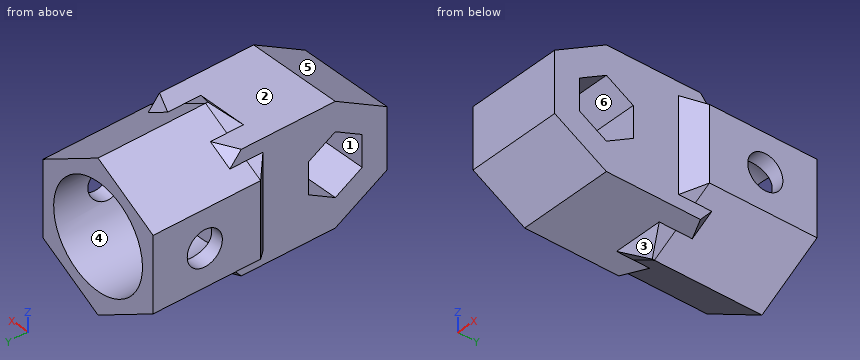
```python
from build123d import *

# Parameters (mm, degrees)
SALIENTE_EXTRUIR1_DEPTH      = 4.6
SALIENTE_EXTRUIR1_DEPTH_BACK = 4.6
SALIENTE_EXTRUIR2_START      = 4
CROQUIS2_R                   = 5
SALIENTE_EXTRUIR2_DEPTH      = 10
CROQUIS4_W                   = 9.2
CROQUIS4_H                   = 2.771281292
SALIENTE_EXTRUIR3_DEPTH      = 9
SALIENTE_EXTRUIR4_START      = 2.6
CROQUIS4_3_W                 = 9.2
CROQUIS4_3_H                 = 6.0044428
SALIENTE_EXTRUIR4_DEPTH      = 6.4
SALIENTE_EXTRUIR5_START      = 3.6
CROQUIS2_2_R                 = 5
SALIENTE_EXTRUIR5_DEPTH      = 0.4
CHAFL_N1_SIZE                = 1.2
CHAFL_N2_SIZE                = 1.6
CROQUIS5_R                   = 1.7
CORTAR_EXTRUIR1_DEPTH        = 24.791034726


with BuildPart() as part:
    # Croquis1 → Saliente-Extruir1 (new, two sides: drawn at the far end of the back side and taken through both)
    with BuildSketch(Plane(origin=(0, 0, 0), x_dir=(0, 0, -1), z_dir=(1, 0, 0)).offset(-SALIENTE_EXTRUIR1_DEPTH_BACK)):
        Polygon((2.886751346, 5), (-2.886751346, 5), (-5.773502692, 0), (-2.886751346, -5), (2.886751346, -5), (5.773502692, 0), align=None)
        Polygon((3.0022214, 0), (1.5011107, 2.6), (-1.5011107, 2.6), (-3.0022214, 0), (-1.5011107, -2.6), (1.5011107, -2.6), align=None, mode=Mode.SUBTRACT)
    extrude(amount=SALIENTE_EXTRUIR1_DEPTH + SALIENTE_EXTRUIR1_DEPTH_BACK)



with BuildPart() as body_2:
    # Croquis2 → Saliente-Extruir2 (new body)
    with BuildSketch(Plane(origin=(0, 5, 0), x_dir=(1, 0, 0), z_dir=(0, 1, 0)).offset(SALIENTE_EXTRUIR2_START)):
        Polygon((0, 7.159143338), (-6.2, 3.579571669), (-6.2, -3.579571669), (0, -7.159143338), (6.2, -3.579571669), (6.2, 3.579571669), align=None)
        with Locations(Location((0, 0, 0), (0, 0, 270))):
            Circle(CROQUIS2_R, mode=Mode.SUBTRACT)
    extrude(amount=SALIENTE_EXTRUIR2_DEPTH)


with BuildPart() as part_1:
    add(part.part)

    add(body_2.part)  # Saliente-Extruir3 merges body 2
    # Croquis4 → Saliente-Extruir3 (add)
    with BuildSketch(Plane(origin=(0, 0, 0), x_dir=(1, 0, 0), z_dir=(0, 1, 0))):
        with Locations((0, -4.387862046)):
            Rectangle(CROQUIS4_W, CROQUIS4_H)
        with Locations((0, 4.387862046)):
            Rectangle(CROQUIS4_W, CROQUIS4_H)
    extrude(amount=SALIENTE_EXTRUIR3_DEPTH)

    # Croquis4<3> → Saliente-Extruir4 (add)
    with BuildSketch(Plane(origin=(0, 0, 0), x_dir=(1, 0, 0), z_dir=(0, 1, 0)).offset(SALIENTE_EXTRUIR4_START)):
        Rectangle(CROQUIS4_3_W, CROQUIS4_3_H)
    extrude(amount=SALIENTE_EXTRUIR4_DEPTH)

    # Croquis2<2> → Saliente-Extruir5 (add)
    # profile 1 of 2: a face of its own
    with BuildSketch(Plane(origin=(0, 5, 0), x_dir=(1, 0, 0), z_dir=(0, 1, 0)).offset(SALIENTE_EXTRUIR5_START)):
        Polygon((6.2, -3.579571669), (6.2, 3.579571669), (0, 7.159143338), (-6.2, 3.579571669), (-6.2, -3.579571669), (0, -7.159143338), align=None)
        with Locations(Location((0, 0, 0), (0, 0, 270))):
            Circle(CROQUIS2_2_R, mode=Mode.SUBTRACT)
    # profile 2 of 2: a face of its own
    with BuildSketch(Plane(origin=(0, 5, 0), x_dir=(1, 0, 0), z_dir=(0, 1, 0)).offset(SALIENTE_EXTRUIR5_START)):
        with Locations(Location((0, 0, 0), (0, 0, 270))):
            Circle(CROQUIS2_2_R)
    extrude(amount=SALIENTE_EXTRUIR5_DEPTH)

    # Chaflán1
    # the kernel refuses this chamfer: 1.2 mm, written as the material it adds along each edge
    with BuildSketch(Plane(origin=(-0.272571358, 9, 7.316512485), x_dir=(0.49981095845564805, -0.027495876610585935, 0.8656979742248805), z_dir=(0.8660254037844388, 0, -0.49999999999999967))) as chafl_n1_piece_1_section:
        Polygon((CHAFL_N1_SIZE * 0.999621916911, -CHAFL_N1_SIZE * 0.0274958766106), (-CHAFL_N1_SIZE * 0.0274958766106, -CHAFL_N1_SIZE * 0.999621916911), (0, 0), align=None)
    chafl_n1_piece_1 = extrude(amount=8.712380356, mode=Mode.PRIVATE)
    chafl_n1_piece_1 = split(chafl_n1_piece_1, bisect_by=Plane(origin=(4.6, 9.457, 5.303539573), z_dir=(-1, 0, 0)), keep=Keep.TOP, mode=Mode.PRIVATE)
    chafl_n1_piece_1 = split(chafl_n1_piece_1, bisect_by=Plane(origin=(3.786, 9.457, 5.773502692), z_dir=(0, 0, -1)), keep=Keep.TOP, mode=Mode.PRIVATE)
    add(chafl_n1_piece_1)
    with BuildSketch(Plane(origin=(-7.272571358, 9, 2.960322307), x_dir=(-0.4998109584556484, -0.027495876610585918, 0.8656979742248802), z_dir=(0.8660254037844387, 0, 0.5000000000000001))) as chafl_n1_piece_2_section:
        Polygon((CHAFL_N1_SIZE * 0.999621916911, -CHAFL_N1_SIZE * 0.0274958766106), (-CHAFL_N1_SIZE * 0.0274958766106, -CHAFL_N1_SIZE * 0.999621916911), (0, 0), align=None)
    chafl_n1_piece_2 = extrude(amount=8.712380356, mode=Mode.PRIVATE)
    chafl_n1_piece_2 = split(chafl_n1_piece_2, bisect_by=Plane(origin=(-4.6, 9.457, 5.303539573), z_dir=(1, 0, 0)), keep=Keep.TOP, mode=Mode.PRIVATE)
    chafl_n1_piece_2 = split(chafl_n1_piece_2, bisect_by=Plane(origin=(-3.786, 9.457, 5.773502692), z_dir=(0, 0, -1)), keep=Keep.TOP, mode=Mode.PRIVATE)
    add(chafl_n1_piece_2)
    with BuildSketch(Plane(origin=(0.272571358, 9, -7.316512485), x_dir=(-0.49981095845564827, -0.027495876610585914, -0.8656979742248804), z_dir=(-0.8660254037844387, 0, 0.49999999999999994))) as chafl_n1_piece_3_section:
        Polygon((CHAFL_N1_SIZE * 0.999621916911, -CHAFL_N1_SIZE * 0.0274958766106), (-CHAFL_N1_SIZE * 0.0274958766106, -CHAFL_N1_SIZE * 0.999621916911), (0, 0), align=None)
    chafl_n1_piece_3 = extrude(amount=8.712380356, mode=Mode.PRIVATE)
    chafl_n1_piece_3 = split(chafl_n1_piece_3, bisect_by=Plane(origin=(-4.6, 9.457, -5.303539573), z_dir=(1, 0, 0)), keep=Keep.TOP, mode=Mode.PRIVATE)
    chafl_n1_piece_3 = split(chafl_n1_piece_3, bisect_by=Plane(origin=(-3.786, 9.457, -5.773502692), z_dir=(0, 0, 1)), keep=Keep.TOP, mode=Mode.PRIVATE)
    add(chafl_n1_piece_3)
    with BuildSketch(Plane(origin=(7.272571358, 9, -2.960322307), x_dir=(-0.013747938305293247, 0.9996219169112968, 0.023812127644090377), z_dir=(-0.8660254037844387, 0, -0.5000000000000001))) as chafl_n1_piece_4_section:
        Polygon((CHAFL_N1_SIZE * 0.999621916911, CHAFL_N1_SIZE * 0.0274958766106), (-CHAFL_N1_SIZE * 0.0274958766106, CHAFL_N1_SIZE * 0.999621916911), (0, 0), align=None)
    chafl_n1_piece_4 = extrude(amount=8.712380356, mode=Mode.PRIVATE)
    chafl_n1_piece_4 = split(chafl_n1_piece_4, bisect_by=Plane(origin=(4.6, 9.457, -5.303539573), z_dir=(-1, 0, 0)), keep=Keep.TOP, mode=Mode.PRIVATE)
    chafl_n1_piece_4 = split(chafl_n1_piece_4, bisect_by=Plane(origin=(3.786, 9.457, -5.773502692), z_dir=(0, 0, 1)), keep=Keep.TOP, mode=Mode.PRIVATE)
    add(chafl_n1_piece_4)

    # Chaflán2
    # the kernel refuses this chamfer: 1.6 mm, written as the material it adds along each edge
    with BuildSketch(Plane(origin=(4.6, 8.6, -8.61802488), x_dir=(0.9996219169112968, 0.027495876610586285, 0), z_dir=(0, 0, 1))) as chafl_n2_piece_1_section:
        Polygon((CHAFL_N2_SIZE * 0.999621916911, -CHAFL_N2_SIZE * 0.0274958766106), (-CHAFL_N2_SIZE * 0.0274958766106, -CHAFL_N2_SIZE * 0.999621916911), (0, 0), align=None)
    chafl_n2_piece_1 = extrude(amount=17.236049761, mode=Mode.PRIVATE)
    chafl_n2_piece_1 = split(chafl_n2_piece_1, bisect_by=Plane(origin=(6.927780638, 8.059532411, -3.159387322), z_dir=(-0.5000000000000001, 0, 0.8660254037844387)), keep=Keep.TOP, mode=Mode.PRIVATE)
    chafl_n2_piece_1 = split(chafl_n2_piece_1, bisect_by=Plane(origin=(6.927780638, 8.059532411, 3.159387322), z_dir=(-0.49999999999999967, 0, -0.8660254037844388)), keep=Keep.TOP, mode=Mode.PRIVATE)
    chafl_n2_piece_1 = split(chafl_n2_piece_1, bisect_by=Plane(origin=(6.2, 8.059532411, 0), z_dir=(-1, 0, 0)), keep=Keep.TOP, mode=Mode.PRIVATE)
    add(chafl_n2_piece_1)
    with BuildSketch(Plane(origin=(-6.514692781, 8.6, -5.773502692), x_dir=(0, 0.027495876610586265, -0.9996219169112966), z_dir=(1, 0, 0))) as chafl_n2_piece_2_section:
        Polygon((CHAFL_N2_SIZE * 0.999621916911, -CHAFL_N2_SIZE * 0.0274958766106), (-CHAFL_N2_SIZE * 0.0274958766106, -CHAFL_N2_SIZE * 0.999621916911), (0, 0), align=None)
    chafl_n2_piece_2 = extrude(amount=13.029385561, mode=Mode.PRIVATE)
    chafl_n2_piece_2 = split(chafl_n2_piece_2, bisect_by=Plane(origin=(0.451958261, 7.972982249, -6.898205114), z_dir=(-0.5000000000000001, 0, 0.8660254037844387)), keep=Keep.TOP, mode=Mode.PRIVATE)
    chafl_n2_piece_2 = split(chafl_n2_piece_2, bisect_by=Plane(origin=(-0.451958261, 7.972982249, -6.898205114), z_dir=(0.49999999999999994, 0, 0.8660254037844387)), keep=Keep.TOP, mode=Mode.PRIVATE)
    add(chafl_n2_piece_2)
    with BuildSketch(Plane(origin=(-4.6, 8.6, -8.61802488), x_dir=(0.027495876610586285, -0.9996219169112968, 0), z_dir=(0, 0, 1))) as chafl_n2_piece_3_section:
        Polygon((CHAFL_N2_SIZE * 0.999621916911, -CHAFL_N2_SIZE * 0.0274958766106), (-CHAFL_N2_SIZE * 0.0274958766106, -CHAFL_N2_SIZE * 0.999621916911), (0, 0), align=None)
    chafl_n2_piece_3 = extrude(amount=17.236049761, mode=Mode.PRIVATE)
    chafl_n2_piece_3 = split(chafl_n2_piece_3, bisect_by=Plane(origin=(-6.927780638, 8.059532411, -3.159387322), z_dir=(0.49999999999999994, 0, 0.8660254037844387)), keep=Keep.TOP, mode=Mode.PRIVATE)
    chafl_n2_piece_3 = split(chafl_n2_piece_3, bisect_by=Plane(origin=(-6.927780638, 8.059532411, 3.159387322), z_dir=(0.5000000000000001, 0, -0.8660254037844387)), keep=Keep.TOP, mode=Mode.PRIVATE)
    chafl_n2_piece_3 = split(chafl_n2_piece_3, bisect_by=Plane(origin=(-6.2, 8.059532411, 0), z_dir=(1, 0, 0)), keep=Keep.TOP, mode=Mode.PRIVATE)
    add(chafl_n2_piece_3)
    with BuildSketch(Plane(origin=(-6.514692781, 8.6, 5.773502692), x_dir=(0, 0.027495876610586265, 0.9996219169112966), z_dir=(1, 0, 0))) as chafl_n2_piece_4_section:
        Polygon((CHAFL_N2_SIZE * 0.999621916911, CHAFL_N2_SIZE * 0.0274958766106), (-CHAFL_N2_SIZE * 0.0274958766106, CHAFL_N2_SIZE * 0.999621916911), (0, 0), align=None)
    chafl_n2_piece_4 = extrude(amount=13.029385561, mode=Mode.PRIVATE)
    chafl_n2_piece_4 = split(chafl_n2_piece_4, bisect_by=Plane(origin=(0.451958261, 7.972982249, 6.898205114), z_dir=(-0.49999999999999967, 0, -0.8660254037844388)), keep=Keep.TOP, mode=Mode.PRIVATE)
    chafl_n2_piece_4 = split(chafl_n2_piece_4, bisect_by=Plane(origin=(-0.451958261, 7.972982249, 6.898205114), z_dir=(0.5000000000000001, 0, -0.8660254037844387)), keep=Keep.TOP, mode=Mode.PRIVATE)
    add(chafl_n2_piece_4)

    # Croquis5 → Cortar-Extruir1 (cut, through all)
    with BuildSketch(Plane(origin=(6.2, 0, 0), x_dir=(0, 0, -1), z_dir=(1, 0, 0))):
        with Locations((0, 14)):
            Circle(CROQUIS5_R)
    extrude(amount=-CORTAR_EXTRUIR1_DEPTH, mode=Mode.SUBTRACT)


solid = part_1.part
```
Part model, mm, in its own coordinate system. Face numbers are marked on the shaded views. A direction names the side the tool comes from. Round coordinates to 2 decimals unless told otherwise and drop trailing zeros. Loops run counter-clockwise (first coordinate to the right, second up) from the corner with the lowest first, then second, coordinate; pieces in that order, holes last.
1. 3-axis set-ups, long thin cutter, end or side, ignore diameter. For the marked faces 4, 5 and 6: which of +Z, -Z, +X, -X, +Y, -Y reach the whole face in a straight line?
Solutions:
face 4: +Y
face 5: +Z, +X, -X, -Y
face 6: +X, -X
2. Slice it at C-C (x = -0.75). Give the cut face in (y, z), and give its area (3 significant figures).
Solutions:
outline: (-5, -2.89) - (0, -5.77) - (7, -5.77) - (7.95, -6.73) - (19, -6.73) - (19, -4.94) - (9, -4.94) - (9, 4.94) - (19, 4.94) - (19, 6.73) - (7.95, 6.73) - (7, 5.77) - (0, 5.77) - (-5, 2.89) - close; hole (-2.6, -1.5) - (0, -3) - (2.6, -1.5) - (2.6, 1.5) - (0, 3) - (-2.6, 1.5) - close
area: 162 mm2
3. Slice it at B-B (z = 0). Give the cut face in (x, y), and give its area (3 significant figures).
Solutions:
outline: (-6.2, 8.6) - (-4.6, 7) - (-4.6, 2.6) - (4.6, 2.6) - (4.6, 7) - (6.2, 8.6) - (6.2, 12.3) - (5, 12.3) - (5, 9) - (-5, 9) - (-5, 12.3) - (-6.2, 12.3) - close; (-6.2, 15.7) - (-5, 15.7) - (-5, 19) - (-6.2, 19) - close; (-4.6, -5) - (4.6, -5) - (4.6, -2.6) - (-4.6, -2.6) - close; (5, 15.7) - (6.2, 15.7) - (6.2, 19) - (5, 19) - close
area: 101 mm2
4. Slice it at D-D (x = 0.5). Give the cut face in (y, z).
Solutions:
outline: (-5, -2.89) - (0, -5.77) - (7, -5.77) - (8.1, -6.87) - (19, -6.87) - (19, -4.97) - (9, -4.97) - (9, 4.97) - (19, 4.97) - (19, 6.87) - (8.1, 6.87) - (7, 5.77) - (0, 5.77) - (-5, 2.89) - close; hole (-2.6, -1.5) - (0, -3) - (2.6, -1.5) - (2.6, 1.5) - (0, 3) - (-2.6, 1.5) - close
5. Two-plate mould, pull along Y, no slides. Class the marked faces 1, 2 and 3: pulls with the +Y half, pulls with the -Y half, needs draft (parallel to the pull), parting line crosses it, or undercut.
Solutions:
face 1: undercut
face 2: needs draft
face 3: pulls with the -Y half
6. Drill centre lines: line 1 along X through (y, z) = (11.75, 0); line 2 along Y through (x, z) = (-1.75, -2.75); line 3 along X through (y, z) = (0.25, 5.5). Where is each one in solid material? Low to high.
Solutions:
line 1: x = -6.2 to -5, 5 to 6.2
line 2: y = -5 to -0.44, 0.44 to 9
line 3: x = -4.6 to 4.6
7. Slice it at A-A (y = 14). Give the cut face in (x, z), and give its area (3 significant figures).
Solutions:
outline: (-6.2, -3.58) - (0, -7.16) - (6.2, -3.58) - (6.2, -1.7) - (4.7, -1.7) arc R5 cw to (-4.7, -1.7) - (-6.2, -1.7) - close; (-6.2, 1.7) - (-4.7, 1.7) arc R5 cw to (4.7, 1.7) - (6.2, 1.7) - (6.2, 3.58) - (0, 7.16) - (-6.2, 3.58) - close
area: 45.8 mm2
8. Flat gauge pins, fed straight in: pin 1 (4 mm diameter, centred on y = 1.5, z = -2.5, fed in from -X); pin 2 (1 mm diameter, centred on x = 4.5, z = 5, fed in from -Y); pin 3 (3 mm diameter, centred on x = 1.5, z = -1, fed in from +Y). Where does each tip first touch, or does it go through?
Solutions:
pin 1: stops at x = -4.6
pin 2: stops at y = -2.21
pin 3: stops at y = 9
